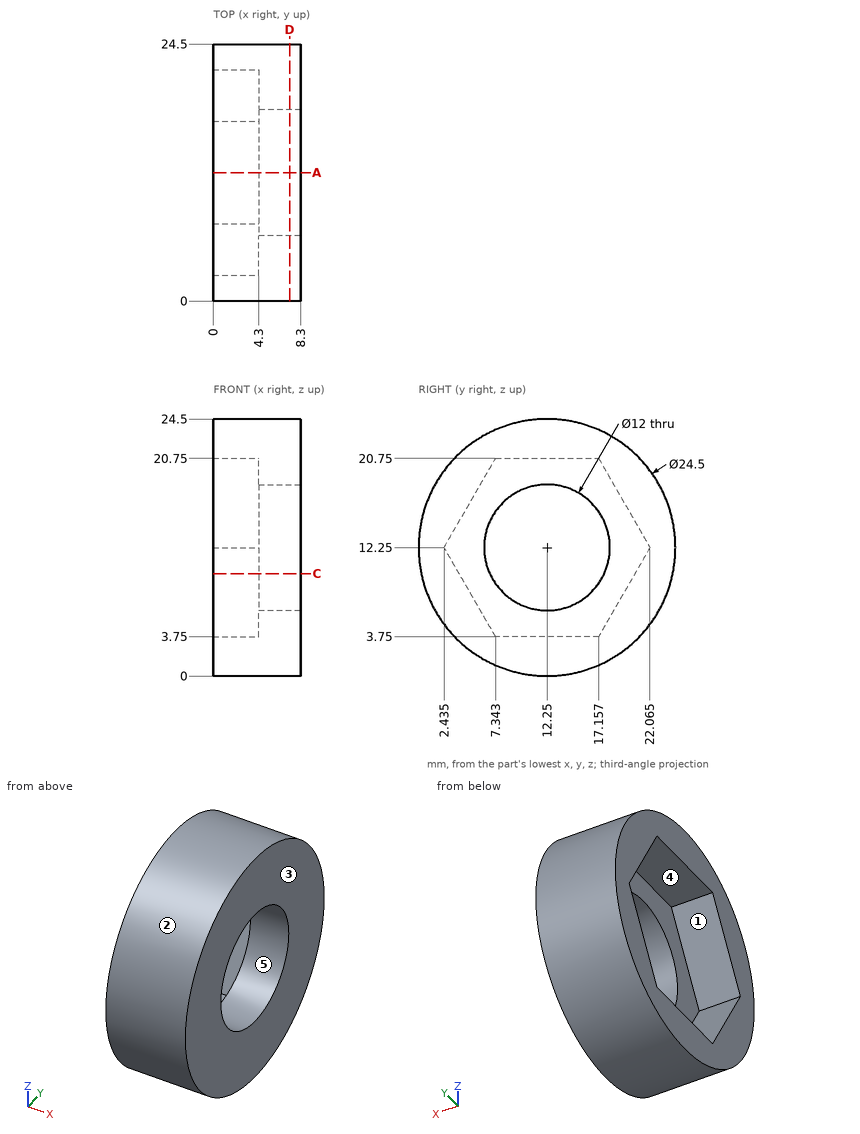
Source: three-view drawing plus pictorial views. Frame: mm from the lowest corner of the part. A direction names the side the tool comes from. Coordinates: 2 decimals unless noted, no trailing zeros. Loops run counter-clockwise (first coordinate to the right, second up) from the corner with the lowest first, then second, coordinate; pieces in that order, holes last. Notation, with made-up numbers: (58, -20.5) - (95, -20.5) arc R16 ccw to (95, 4.5) - close; hole circle Ø6 at (-24, 5.5). An arc over 180 degrees is marked (long way). One line per item, written item: value. Start each with the question number.
1. Section C-C (z = 9.75). Return the cut outline in (x, y) (1 decimal).
2. Ray query, L1, parallel to Z at x = 6.25, y = 12.25; L2, parallel to Y at x = 5.5, z = 14.75 (1 decimal); L3, parallel to Y at x = 2, z = 13 (1 decimal). Return the intervals inside material, ascending.
3. Contact query for flat-ended pins moving along their axis: P1, Ø3, axis at x = 6.5, z = 10, coming from the +Y side; P2, Ø1, axis at x = 4, z = 10, coming from the -Y side (1 decimal). Output: stop coordinate, or through.
4. Section D-D (x = 7.25). Return the cut outline in (y, z), and give its area (3 significant figures).
5. Mould query, pull axis Y, two halves, no side actions, for the marked faces 1, 2 and 3. Classes: pulls with the +Y half, pulls with the -Y half, needs draft (parallel to the pull), parting line crosses it, or undercut.
6. Section A-A (y = 12.25). Return the cut outline in (x, z).
7. Set-up query: the marked faces 4 and 5. Return all of +Z, -Z, +X, -X, +Y, -Y with unobstructed straight access to the full face (end or side cutting, diameter ignored); none if empty.
Verdict:
1. outline: (0, 0.3) - (8.3, 0.3) - (8.3, 6.8) - (4.3, 6.8) - (4.3, 3.9) - (0, 3.9) - close; (0, 20.6) - (4.3, 20.6) - (4.3, 17.7) - (8.3, 17.7) - (8.3, 24.2) - (0, 24.2) - close
2. L1: z = 0 to 6.25, 18.25 to 24.5
2. L2: y = 0.3 to 6.8, 17.7 to 24.2
2. L3: y = 0 to 2.9, 21.6 to 24.5
3. P1: stops at y = 24.48
3. P2: stops at y = 0.1
4. outline: circle Ø24.5 at (12.25, 12.25); hole circle Ø12 at (12.25, 12.25)
4. area: 358 mm2
5. face 1: undercut
5. face 2: parting line crosses it
5. face 3: needs draft
6. outline: (0, 0) - (8.3, 0) - (8.3, 6.25) - (4.3, 6.25) - (4.3, 3.75) - (0, 3.75) - close; (0, 20.75) - (4.3, 20.75) - (4.3, 18.25) - (8.3, 18.25) - (8.3, 24.5) - (0, 24.5) - close
7. face 4: -X
7. face 5: +X, -X
